```python
from build123d import *

# Parameters (mm, degrees)
SKETCH1_W           = 203.2
SKETCH1_H           = 25.4
BOSS_EXTRUDE1_DEPTH = 6.35
SKETCH2_R           = 4.7625
CUT_EXTRUDE1_DEPTH  = 7.35
LPATTERN1_COUNT     = 4
LPATTERN1_PITCH     = 50.8


with BuildPart() as part:
    # Sketch1 → Boss-Extrude1 (new body)
    with BuildSketch(Plane.XY):
        Rectangle(SKETCH1_W, SKETCH1_H)
    extrude(amount=BOSS_EXTRUDE1_DEPTH)

    # Sketch2 → Cut-Extrude1 (cut, through all)
    with BuildSketch(Plane.XY.offset(6.35)):
        with Locations((-76.2, 0)):
            Circle(SKETCH2_R)
    cut_extrude1 = extrude(amount=-CUT_EXTRUDE1_DEPTH, mode=Mode.SUBTRACT)

    # LPattern1: Cut-Extrude1 ×4
    with Locations(*[(i * LPATTERN1_PITCH, 0, 0) for i in range(1, LPATTERN1_COUNT)]):
        add(cut_extrude1, mode=Mode.SUBTRACT)


solid = part.part
```
Design review of the part built by this model. Coordinates are the model's own, in mm. Coordinates: 2 decimals unless noted, no trailing zeros. Loops run counter-clockwise (first coordinate to the right, second up) from the corner with the lowest first, then second, coordinate; pieces in that order, holes last. Notation, with made-up numbers: (-8, 36) -> (5, 36) arc R16 ccw to (5, 43) -> close; hole circle Ø8 at (19, 5). An arc over 180 degrees is marked (long way). Answer as a JSON object with one key per item and string values.
Q1. Take a section at A-A on y = 0. Give the boundary of the cut face in (x, z).
Answer block:
{"outline": "(-101.6, 0) -> (-80.96, 0) -> (-80.96, 6.35) -> (-101.6, 6.35) -> close; (-71.44, 0) -> (-30.16, 0) -> (-30.16, 6.35) -> (-71.44, 6.35) -> close; (-20.64, 0) -> (20.64, 0) -> (20.64, 6.35) -> (-20.64, 6.35) -> close; (30.16, 0) -> (71.44, 0) -> (71.44, 6.35) -> (30.16, 6.35) -> close; (80.96, 0) -> (101.6, 0) -> (101.6, 6.35) -> (80.96, 6.35) -> close"}
Q2. Clearance check with a flat-ended pin moving along its axis: pin 1 Ø15 at (x, y) = (-25.4, 0) entering from -Z. State where the tip first meets the part, or that it passes through.
Answer block:
{"pin 1": "stops at z = 0"}
Q3. To check wall thickness, follow L1, parallel to Y at x = 25.4, z = 3.5; L2, parallel to X at y = 3.5, z = 0.75; L3, parallel to Y at x = 26, z = 1.25. State the ranges of each line that lie inside material, in increasing order.
Answer block:
{"L1": "y = -12.7 to -4.76, 4.76 to 12.7", "L2": "x = -101.6 to -79.43, -72.97 to -28.63, -22.17 to 22.17, 28.63 to 72.97, 79.43 to 101.6", "L3": "y = -12.7 to -4.72, 4.72 to 12.7"}
Q4. Take a section at C-C on z = 5. Give the boundary of the cut face in (x, y) (1 decimal).
Answer block:
{"outline": "(-101.6, -12.7) -> (101.6, -12.7) -> (101.6, 12.7) -> (-101.6, 12.7) -> close; hole circle Ø9.5 at (-76.2, 0); hole circle Ø9.5 at (-25.4, 0); hole circle Ø9.5 at (25.4, 0); hole circle Ø9.5 at (76.2, 0)"}
Q5. The part is to be moulded in two halves that separate along Y. For faces 1 (the cylindrical face through (-80.958, 0.209, 3.219)), 2 (the flat face through (-1, 0, 6.35)), 3 (the cylindrical face through (21.62, -2.9, 3.22)), 4 (the flat face through (-1, 12.7, 3)), say which applies: +Y half, -Y half, draft (parallel to the pull), parting line (faces both ways), or undercut.
Answer block:
{"face 1": "undercut", "face 2": "draft", "face 3": "undercut", "face 4": "+Y half"}
Q6. Take a section at B-B on x = 25.4. Give the boundary of the cut face in (y, z), plus the area to 3 significant figures.
Answer block:
{"outline": "(-12.7, 0) -> (-4.76, 0) -> (-4.76, 6.35) -> (-12.7, 6.35) -> close; (4.76, 0) -> (12.7, 0) -> (12.7, 6.35) -> (4.76, 6.35) -> close", "area": "101 mm^2"}
